Read the model definition and answer for the solid it produces. Units are mm, in the model's axes. Face numbers are marked on the shaded views. A direction names the side the tool comes from. Give positions to 0.01 mm unless a question says otherwise; leave off trailing zeros. Write each loop counter-clockwise with the first axis right and the second up, starting at its lowest first coordinate (ties: lowest second). Pieces come first, ordered by that corner, then holes. Notation, with made-up numbers: (79.25, 50.25) - (129.25, 50.25) arc R14 ccw to (129.25, 60.25) - close; hole circle Ø10 at (17.5, 26.25). An arc over 180 degrees is marked (long way). Answer as CSV lines item,"result".
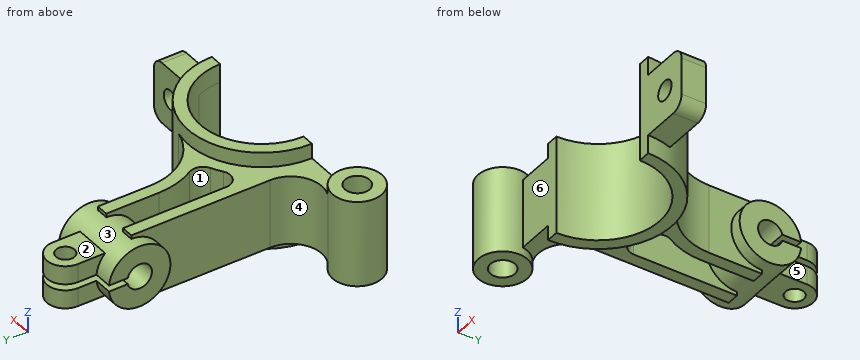
```python
from build123d import *

# Parameters (mm, degrees)
EXTRUDE_THIN1_DEPTH          = 40
SKETCH2_R                    = 20
SKETCH2_R_2                  = 10
EXTRUDE_THIN2_DEPTH          = 35
SKETCH3_W                    = 100
SKETCH3_H                    = 50
BOSS_EXTRUDE1_DEPTH          = 20
DELETEFACE4_START            = -25
DELETEFACE4_DEPTH            = 50
FILLET1_R                    = 10
SKETCH5_W                    = 8
SKETCH5_H                    = 42.929151324
SKETCH6_R                    = 25
BOSS_EXTRUDE2_DEPTH          = 60
SKETCH7_R                    = 7.5
BOSS_EXTRUDE3_DEPTH          = 17.5
BOSS_EXTRUDE4_DEPTH          = 28
F_20_0_20_DIAMETER_HOLE1_D   = 20
CUT_EXTRUDE_THIN1_DEPTH      = 239.432380351
CUT_EXTRUDE_THIN1_DEPTH_BACK = 239.432380351
SKETCH11_W                   = 5
SKETCH11_H                   = 55


# Read off the part's stored shape, not the designer's step: DeleteFace4
with BuildPart() as part:
    # Sketch1 → Extrude-Thin1 (new, symmetric)
    with BuildSketch(Plane.XY):
        with BuildLine():
            ThreePointArc((60, 0), (0, 60), (-60, 0))
            Line((-60, 0), (-50, 0))
            ThreePointArc((-50, 0), (0, 50), (50, 0))
            Line((50, 0), (60, 0))
        make_face()
    extrude(amount=EXTRUDE_THIN1_DEPTH, both=True)

    # Sketch3 → Boss-Extrude1 (add)
    with BuildSketch(Plane.XZ):
        with Locations((50, 0)):
            Rectangle(SKETCH3_W, SKETCH3_H)
    extrude(amount=-BOSS_EXTRUDE1_DEPTH)

    # DeleteFace4 outline → DeleteFace4 (cut)
    with BuildSketch(Plane.XY.offset(DELETEFACE4_START)):
        with BuildLine():
            ThreePointArc((50, 0), (48.945315647, 10.215482184), (45.82575695, 20))
            Line((45.82575695, 20), (0, 20))
            Line((0, 20), (0, 0))
            Line((0, 0), (50, 0))
        make_face()
    extrude(amount=DELETEFACE4_DEPTH, mode=Mode.SUBTRACT)

    # Fillet1
    fillet1_edges = [part.edges().sort_by_distance(p)[0] for p in [
        (100, 10, -25),
        (100, 10, 25),
    ]]
    fillet(fillet1_edges, radius=FILLET1_R)

    # Sketch5 → Ø16.0 (16) Diameter Hole1 (revolve, cut)
    with BuildSketch(Plane(origin=(80, 20, 0), x_dir=(0, 0, 1), z_dir=(1, 0, 0))):
        with Locations((4, 21.464575662)):
            Rectangle(SKETCH5_W, SKETCH5_H)
    revolve(axis=Axis((80, 26.35, 0), (0, -1, 0)), mode=Mode.SUBTRACT)



with BuildPart() as body_2:
    # Sketch2 → Extrude-Thin2 (new, symmetric)
    with BuildSketch(Plane.XY):
        with Locations((-110, -2.929151324)):
            Circle(SKETCH2_R)
        with Locations((-110, -2.929151324)):
            Circle(SKETCH2_R_2, mode=Mode.SUBTRACT)
    extrude(amount=EXTRUDE_THIN2_DEPTH, both=True)


with BuildPart() as body_3:
    # Sketch6 → Boss-Extrude2 (new body)
    with BuildSketch(Plane(origin=(-15, 0, 0), x_dir=(0, 0, -1), z_dir=(1, 0, 0))):
        with Locations((0, 150)):
            Circle(SKETCH6_R)
    extrude(amount=-BOSS_EXTRUDE2_DEPTH)

    # Sketch7 → Boss-Extrude3 (add, symmetric)
    with BuildSketch(Plane.XY):
        with BuildLine():
            Line((-60, 150), (-60, 190))
            ThreePointArc((-60, 190), (-45, 205), (-30, 190))
            Line((-30, 190), (-30, 150))
            Line((-30, 150), (-60, 150))
        make_face()
        with Locations((-45, 190)):
            Circle(SKETCH7_R, mode=Mode.SUBTRACT)
    extrude(amount=BOSS_EXTRUDE3_DEPTH, both=True)


with BuildPart() as part_1:
    add(part.part)

    add(body_2.part)  # Boss-Extrude4 merges body 2

    add(body_3.part)  # Boss-Extrude4 merges body 3
    # Sketch8 → Boss-Extrude4 (add, symmetric)
    with BuildSketch(Plane.XY):
        with BuildLine():
            Line((-25, 150), (-25, 107.121426428))
            ThreePointArc((-25, 107.121426428), (-14.16747259, 76.042348403), (13.636363636, 58.429868961))
            ThreePointArc((13.636363636, 58.429868961), (-37.29489363, 47.000967108), (-60, 0))
            Line((-60, 0), (-90.215660928, 0))
            ThreePointArc((-90.215660928, 0), (-93.823137808, 8.831338871), (-101.111111111, 14.986977006))
            ThreePointArc((-101.111111111, 14.986977006), (-76.823843083, 16.136222778), (-65, 37.382137418))
            Line((-65, 37.382137418), (-65, 150))
            Line((-65, 150), (-55, 150))
            Line((-55, 150), (-55, 66.143782777))
            ThreePointArc((-55, 66.143782777), (-49.677071733, 57.304948012), (-39.375, 57.87580993))
            ThreePointArc((-39.375, 57.87580993), (-35.260419238, 60.470677482), (-30.975558625, 62.773519639))
            ThreePointArc((-30.975558625, 62.773519639), (-25.821810248, 68.869571549), (-26.771975796, 76.79548832))
            ThreePointArc((-26.771975796, 76.79548832), (-32.906470052, 91.410260777), (-35, 107.121426428))
            Line((-35, 107.121426428), (-35, 150))
            Line((-35, 150), (-25, 150))
        make_face()
    extrude(amount=BOSS_EXTRUDE4_DEPTH, both=True)

    # Ø20.0 (20) Diameter Hole1 (through all)
    with Locations(Plane(origin=(-15, 0, 0), x_dir=(0, 0, -1), z_dir=(1, 0, 0))):
        with Locations((0, 150)):
            Hole(F_20_0_20_DIAMETER_HOLE1_D / 2)

    # Sketch11 → Cut-Extrude-Thin1 (cut, two sides: drawn at the far end of the back side and taken through both)
    with BuildSketch(Plane(origin=(-15, 0, 0), x_dir=(0, 0, -1), z_dir=(1, 0, 0)).offset(-CUT_EXTRUDE_THIN1_DEPTH_BACK)):
        with Locations((0, 177.5)):
            Rectangle(SKETCH11_W, SKETCH11_H)
    extrude(amount=CUT_EXTRUDE_THIN1_DEPTH + CUT_EXTRUDE_THIN1_DEPTH_BACK, mode=Mode.SUBTRACT)


solid = part_1.part
```
(1) Each of these flat-tipped pins is pushed along its axis until it touches: P1, Ø16, axis at x = 74, y = 8.5, coming from the +Z side; P2, Ø1.5, axis at x = -32, z = -26.5, coming from the +Y side; P3, Ø21.5, axis at y = 119, z = -6.5, coming from the -X side. Where does it stop, or does it pass through?
Worked out:
P1,"stops at z = 25"
P2,"stops at y = 150"
P3,"stops at x = -75"
(2) A cutting plane is placed at B-B (y = 113.5). Write down the section's boundary in (x, z), and give its area (3 significant figures).
Worked out:
outline,"(-65, -28) - (-55, -28) - (-55, 28) - (-65, 28) - close; (-35, -28) - (-25, -28) - (-25, 28) - (-35, 28) - close"
area,"1,120 mm^2"
(3) For the marked faces 1, 2 and 3, determine the directions among +Z, -Z, +X, -X, +Y, -Y from which every point of the face is accessible in a straight line to the end or side of a thin tool.
Worked out:
face 1,"+Z, -Z"
face 2,"+Z, +X, -X, +Y"
face 3,"none"
(4) A cutting plane is placed at C-C (x = -45). Write down the section's boundary in (y, z).
Worked out:
outline,"(21.79, -40) - (39.69, -40) - (39.69, -28) - (56.14, -28) - (56.14, 28) - (39.69, 28) - (39.69, 40) - (21.79, 40) - close; (159.68, -2.5) arc R10 cw (long way) to (159.68, 2.5) - (182.5, 2.5) - (182.5, 17.5) - (167.85, 17.5) arc R25 ccw (long way) to (167.85, -17.5) - (182.5, -17.5) - (182.5, -2.5) - close; (197.5, -17.5) - (205, -17.5) - (205, -2.5) - (197.5, -2.5) - close; (197.5, 2.5) - (205, 2.5) - (205, 17.5) - (197.5, 17.5) - close"
(5) The mould has two halves that part along X. Classify the marked faces 4, 5 and 6: +X half, -X half, draft (parallel to the pull), parting line (faces both ways), or undercut.
Worked out:
face 4,"undercut"
face 5,"+X half"
face 6,"draft"
(6) Find the intervals of material crossed by L1, parallel to Z at x = 80, y = 9; L2, parallel to X at y = 120, z = -21; L3, parallel to Y at x = 62, z = -0.5, in increasing order.
Worked out:
L1,"z = -25 to -8, 8 to 25"
L2,"x = -65 to -55, -35 to -25"
L3,"y = 0 to 20"
(7) A cutting plane is placed at A-A (x = -110). Write down the section's boundary in (y, z).
Worked out:
outline,"(-22.93, -35) - (-12.93, -35) - (-12.93, 35) - (-22.93, 35) - close; (7.07, -35) - (17.07, -35) - (17.07, 35) - (7.07, 35) - close"
(8) A cutting plane is placed at D-D (x = -4.5). Write down the section's boundary in (y, z).
Worked out:
outline,"(49.8, -40) - (59.83, -40) - (59.83, -28) - (66.75, -28) - (66.75, 28) - (59.83, 28) - (59.83, 40) - (49.8, 40) - close"
